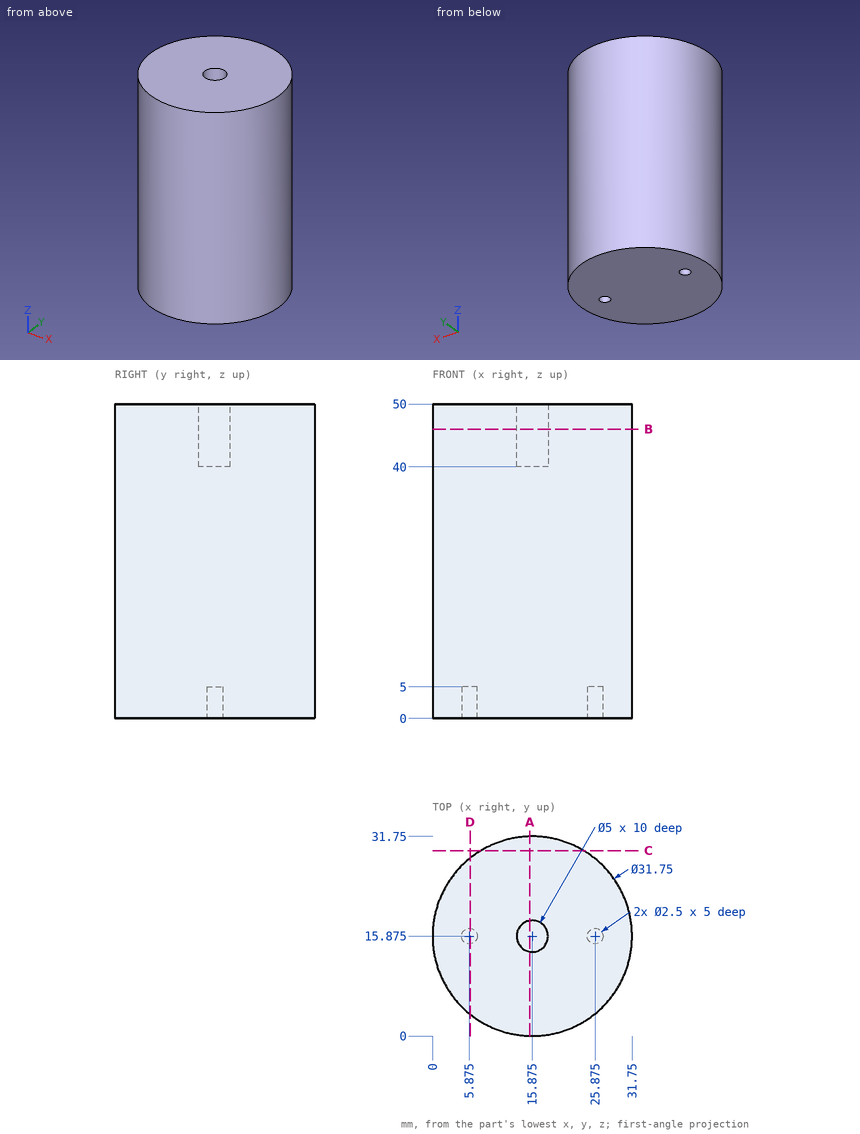
Answer from the drawing. Dimensions are ordinates in mm from the lowest x, y and z of the part. Give positions to 0.01 mm unless a question says otherwise; leave off trailing zeros. Loops run counter-clockwise (first coordinate to the right, second up) from the corner with the lowest first, then second, coordinate; pieces in that order, holes last. Notation, with made-up numbers: (11, -27.5) - (45, -27.5) arc R34 ccw to (45, 9.5) - close; hole circle Ø9 at (69.25, 87). An arc over 180 degrees is marked (long way). Answer as a JSON object with one key per item and string values.
1. A cutting plane is placed at C-C (y = 29.5). Write down the section's boundary in (x, z).
Determined:
{"outline": "(7.73, 0) - (24.02, 0) - (24.02, 50) - (7.73, 50) - close"}
2. A cutting plane is placed at B-B (z = 46). Write down the section's boundary in (x, y) (3 decimals), then the cut area to 3 significant figures.
Determined:
{"outline": "circle Ø31.75 at (15.875, 15.875); hole circle Ø5 at (15.875, 15.875)", "area": "772 mm²"}
3. A cutting plane is placed at D-D (x = 6). Write down the section's boundary in (y, z), then the cut area to 3 significant figures.
Determined:
{"outline": "(3.45, 0) - (14.63, 0) - (14.63, 5) - (17.12, 5) - (17.12, 0) - (28.3, 0) - (28.3, 50) - (3.45, 50) - close", "area": "1,230 mm²"}
4. Flat-ended cylindrical pins translate along their axes: pin 1 Ø0.8 at (x, y) = (5.5, 15.5) entering from -Z; pin 2 Ø1 at (x, z) = (21, 9.5) entering from -Y; pin 3 Ø4 at (y, z) = (7.5, 20.5) entering from +X. Find the tip coordinate at first contact, or state that the pin passes through.
Determined:
{"pin 1": "z = 5", "pin 2": "y = 0.69", "pin 3": "x = 30.41"}
5. A cutting plane is placed at A-A (x = 15.5). Write down the section's boundary in (y, z), then the cut area to 3 significant figures.
Determined:
{"outline": "(0, 0) - (31.75, 0) - (31.75, 50) - (18.35, 50) - (18.35, 40) - (13.4, 40) - (13.4, 50) - (0, 50) - close", "area": "1,540 mm²"}
6. Find the intervals of material crossed by L1, parallel to Y at x = 16, z = 48; L2, parallel to X at y = 16, z = 11.5; L3, parallel to Y at x = 11, z = 9, in increasing order. Write a range as [from, to].
Determined:
{"L1": "[0, 13.38], [18.37, 31.75]", "L2": "[0, 31.75]", "L3": "[0.77, 30.98]"}
